```python
from build123d import *

# Parameters (mm, degrees)
SKETCH_1_R      = 3.55
SKETCH_1_W      = 7
SKETCH_1_H      = 7
EXTRUDE_1_DEPTH = 100
FILLET_1_R      = 1
FILLET_2_R      = 2.5


with BuildPart() as part:
    # 草图1 → 凸台-拉伸1 (new body)
    with BuildSketch(Plane(origin=(0, 0, 0), x_dir=(1, 0, 0), z_dir=(0, 1, 0))):
        Polygon((-20, 20), (-4.25, 20), (-4.25, 18.2), (-10, 18.2), (-10, 11.343502884), (-3.956497116, 5.3), (3.956497116, 5.3), (10, 11.343502884), (10, 18.2), (4.25, 18.2), (4.25, 20), (20, 20), (20, 4.25), (18.2, 4.25), (18.2, 10), (11.343502884, 10), (5.3, 3.956497116), (5.3, -3.956497116), (11.343502884, -10), (18.2, -10), (18.2, -4.25), (20, -4.25), (20, -20), (4.25, -20), (4.25, -18.2), (10, -18.2), (10, -11.343502884), (3.956497116, -5.3), (-3.956497116, -5.3), (-10, -11.343502884), (-10, -18.2), (-4.25, -18.2), (-4.25, -20), (-20, -20), (-20, -4.25), (-18.2, -4.25), (-18.2, -10), (-11.343502884, -10), (-5.3, -3.956497116), (-5.3, 3.956497116), (-11.343502884, 10), (-18.2, 10), (-18.2, 4.25), (-20, 4.25), align=None)
        with Locations(Location((0, 0, 0), (0, 0, 270))):
            Circle(SKETCH_1_R, mode=Mode.SUBTRACT)
        with Locations((-15, 15)):
            Rectangle(SKETCH_1_W, SKETCH_1_H, mode=Mode.SUBTRACT)
        with Locations((15, 15)):
            Rectangle(SKETCH_1_W, SKETCH_1_H, mode=Mode.SUBTRACT)
        with Locations((15, -15)):
            Rectangle(SKETCH_1_W, SKETCH_1_H, mode=Mode.SUBTRACT)
        with Locations((-15, -15)):
            Rectangle(SKETCH_1_W, SKETCH_1_H, mode=Mode.SUBTRACT)
    extrude(amount=EXTRUDE_1_DEPTH)

    # 圆角1
    fillet_1_edges = [part.edges().sort_by_distance(p)[0] for p in [
        (-18.5, 50, -18.5),
        (18.5, 50, -18.5),
        (18.5, 50, 18.5),
        (-18.5, 50, 18.5),
    ]]
    fillet(fillet_1_edges, radius=FILLET_1_R)

    # 圆角2
    fillet_2_edges = [part.edges().sort_by_distance(p)[0] for p in [
        (-20, 50, -20),
        (20, 50, -20),
        (20, 50, 20),
        (-20, 50, 20),
    ]]
    fillet(fillet_2_edges, radius=FILLET_2_R)


solid = part.part
```
Source: CAD feature listing. Evaluate the final solid. Frame: model axes, mm. A direction names the side the tool comes from. Coordinates: 2 decimals unless noted, no trailing zeros. Write each loop counter-clockwise with the first axis right and the second up, starting at its lowest first coordinate (ties: lowest second). Pieces come first, ordered by that corner, then holes. Notation, with made-up numbers: (-16.75, 29) -> (6.25, 29) arc R29 cw to (6.25, 59) -> close; hole circle Ø6 at (-35, 4). An arc over 180 degrees is marked (long way). Return JSON: item names as keys, results as strings. Group by question number.
1) Set-up query: faces 1 (the face through (20, 49, 11)), 2 (the face through (19, 49, -4.25)), 3 (the face through (-19, 49, -4.25)), 4 (the face through (-7.021, 49.3, -8.364)). Return all of +Z, -Z, +X, -X, +Y, -Y with unobstructed straight access to the full face (end or side cutting, diameter ignored); none if empty.
2) Mould query, pull axis Z, two halves, no side actions, for faces 5 (the face through (7, 49, -18.2)), 6 (the face through (-11, 49, -20)), 7 (the face through (19.287, 50.7, 19.248)). Classes: +Z half, -Z half, draft (parallel to the pull), parting line (faces both ways), or undercut.
3) Ray query, line 1 along X through (y, z) = (82.5, -14.5); line 2 along X through (y, z) = (61.5, 7.5). Return the intervals inside material, ascending.
4) Contact query for flat-ended pins moving along their axis: P1, Ø1, axis at y = 68.5, z = -3.5, coming from the +X side; P2, Ø2, axis at y = 43, z = -19, coming from the -X side; P3, Ø1.4, axis at y = 43, z = 19, coming from the +X side. Output: stop coordinate, or through.
5) Section query C-C, the plane z = 0. Return loops of the section in (x, y), plus the area to 3 significant figures.
6) Section query A-A, the plane z = 16.5. Return loops of the section in (x, y).
7) Section query B-B, the plane x = 0. Return loops of the section in (y, z).
8) Section query D-D, the plane x = -13. Return loops of the section in (y, z), plus the area to 3 significant figures.
From the geometry:
{
 "1": {"face 1": "+Z, -Z, +X, +Y, -Y", "face 2": "+X, +Y, -Y", "face 3": "-X, +Y, -Y", "face 4": "+Y, -Y"},
 "2": {"face 5": "undercut", "face 6": "-Z half", "face 7": "+Z half"},
 "3": {"line 1": "-20 to -18.5, -11.5 to -10, 10 to 11.5, 18.5 to 20", "line 2": "-20 to -18.2, -8.84 to -6.16, 6.16 to 8.84, 18.2 to 20"},
 "4": {"P1": "x = 5.34", "P2": "x = -19.95", "P3": "x = 19.87"},
 "5": {"outline": "(-5.3, 0) -> (-3.55, 0) -> (-3.55, 100) -> (-5.3, 100) -> close; (3.55, 0) -> (5.3, 0) -> (5.3, 100) -> (3.55, 100) -> close", "area": "350 mm²"},
 "6": {"outline": "(-20, 0) -> (-18.5, 0) -> (-18.5, 100) -> (-20, 100) -> close; (-11.5, 0) -> (-10, 0) -> (-10, 100) -> (-11.5, 100) -> close; (10, 0) -> (11.5, 0) -> (11.5, 100) -> (10, 100) -> close; (18.5, 0) -> (20, 0) -> (20, 100) -> (18.5, 100) -> close"},
 "7": {"outline": "(0, -5.3) -> (100, -5.3) -> (100, -3.55) -> (0, -3.55) -> close; (0, 3.55) -> (100, 3.55) -> (100, 5.3) -> (0, 5.3) -> close"},
 "8": {"outline": "(0, -20) -> (100, -20) -> (100, -18.5) -> (0, -18.5) -> close; (0, -11.5) -> (100, -11.5) -> (100, -10) -> (0, -10) -> close; (0, 10) -> (100, 10) -> (100, 11.5) -> (0, 11.5) -> close; (0, 18.5) -> (100, 18.5) -> (100, 20) -> (0, 20) -> close", "area": "600 mm²"}
}
